Check sheet for the modelled part. Datum: model origin and axes. Units: mm. Face numbers are marked on the shaded views. A direction names the side the tool comes from. Give positions to 0.01 mm unless a question says otherwise; leave off trailing zeros. Write each loop counter-clockwise with the first axis right and the second up, starting at its lowest first coordinate (ties: lowest second). Pieces come first, ordered by that corner, then holes. Notation, with made-up numbers: (35.25, 1.25) -> (45.25, 1.25) arc R28 ccw to (45.25, 37.25) -> close; hole circle Ø5 at (74.25, -10). An arc over 180 degrees is marked (long way). Return JSON: item names as keys, results as strings.
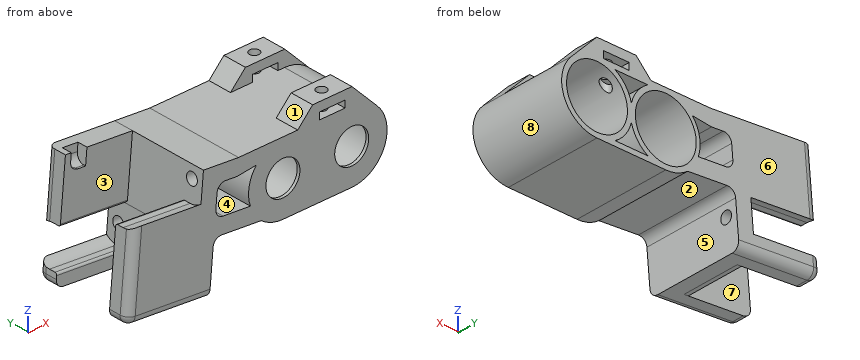
from build123d import *

# Parameters (mm, degrees)
SKETCH1_R               = 7.75
BOSS_EXTRUDE1_DEPTH     = 24
BOSS_EXTRUDE2_START     = 0.75
SKETCH2_R               = 4.33
BOSS_EXTRUDE2_DEPTH     = 0.75
SKETCH4_W               = 10
SKETCH4_H               = 6
BOSS_EXTRUDE4_DEPTH     = 4
CUT_EXTRUDE1_DEPTH      = 35.968736037
CUT_EXTRUDE1_DEPTH_BACK = 35.968736037
SKETCH5_W               = 6.5
SKETCH5_H               = 1.75
SKETCH6_R               = 1.25
CUT_EXTRUDE2_DEPTH      = 16
BOSS_EXTRUDE5_START     = -24.75
BOSS_EXTRUDE5_DEPTH     = 24.75
CUT_EXTRUDE3_DEPTH      = 39.520286863
SKETCH9_W               = 12.886425037
SKETCH9_H               = 24.75
BOSS_EXTRUDE6_DEPTH     = 4
FILLET1_R               = 2
FILLET2_R               = 2
BOSS_EXTRUDE9_DEPTH     = 17.13
SKETCH14_R              = 1.5
CUT_EXTRUDE5_DEPTH      = 6
BOSS_EXTRUDE10_DEPTH    = 14.84
FILLET4_R               = 2
SKETCH16_W              = 4
SKETCH16_H              = 2.5
CUT_EXTRUDE6_DEPTH      = 4
FILLET5_R               = 2
BOSS_EXTRUDE11_DEPTH    = 6
BOSS_EXTRUDE12_START    = -6
BOSS_EXTRUDE12_DEPTH    = 6


with BuildPart() as part:
    # Sketch1 → Boss-Extrude1 (new body)
    with BuildSketch(Plane(origin=(0, 0, 0), x_dir=(1, 0, 0), z_dir=(0, 1, 0))):
        with BuildLine():
            Line((0, -9), (17.5, -9))
            ThreePointArc((17.5, -9), (26.5, 0), (17.5, 9))
            Line((17.5, 9), (0, 9))
            ThreePointArc((0, 9), (-9, 0), (0, -9))
        make_face()
        with Locations(Location((17.5, 0, 0), (0, 0, 270))):
            Circle(SKETCH1_R, mode=Mode.SUBTRACT)
        with BuildLine():
            ThreePointArc((8.75, -2.106537443), (10.26424991, -5.352001554), (12.924248696, -7.75))
            Line((12.924248696, -7.75), (4.575751304, -7.75))
            ThreePointArc((4.575751304, -7.75), (7.23575009, -5.352001554), (8.75, -2.106537443))
        make_face(mode=Mode.SUBTRACT)
        with Locations(Location((0, 0, 0), (0, 0, 270))):
            Circle(SKETCH1_R, mode=Mode.SUBTRACT)
        with BuildLine():
            Line((4.575751304, 7.75), (12.924248696, 7.75))
            ThreePointArc((12.924248696, 7.75), (10.26424991, 5.352001554), (8.75, 2.106537443))
            ThreePointArc((8.75, 2.106537443), (7.23575009, 5.352001554), (4.575751304, 7.75))
        make_face(mode=Mode.SUBTRACT)
    extrude(amount=BOSS_EXTRUDE1_DEPTH)

    # Sketch2 → Boss-Extrude2 (add)
    with BuildSketch(Plane.XZ.offset(BOSS_EXTRUDE2_START)):
        with BuildLine():
            Line((17.5, 9), (0, 9))
            ThreePointArc((0, 9), (-9, 0), (0, -9))
            Line((0, -9), (17.5, -9))
            ThreePointArc((17.5, -9), (26.5, 0), (17.5, 9))
        make_face()
        with Locations(Location((17.5, 0, 0), (0, 0, 270))):
            Circle(SKETCH2_R, mode=Mode.SUBTRACT)
        with Locations(Location((0, 0, 0), (0, 0, 270))):
            Circle(SKETCH2_R, mode=Mode.SUBTRACT)
    extrude(amount=-BOSS_EXTRUDE2_DEPTH)

    # Sketch4 → Boss-Extrude4 (add)
    with BuildSketch(Plane.XY.offset(9)):
        with Locations((12.5625, 2.25)):
            Rectangle(SKETCH4_W, SKETCH4_H)
        with Locations((12.5625, 21)):
            Rectangle(SKETCH4_W, SKETCH4_H)
    extrude(amount=BOSS_EXTRUDE4_DEPTH)

    # Sketch5 → Cut-Extrude1 (cut, two sides: drawn at the far end of the back side and taken through both)
    with BuildSketch(Plane.XZ.offset(-18).offset(-CUT_EXTRUDE1_DEPTH_BACK)):
        with Locations((12.5625, 9.875)):
            Rectangle(SKETCH5_W, SKETCH5_H)
    extrude(amount=CUT_EXTRUDE1_DEPTH + CUT_EXTRUDE1_DEPTH_BACK, mode=Mode.SUBTRACT)

    # Sketch6 → Cut-Extrude2 (cut)
    with BuildSketch(Plane.XY.offset(13)):
        with Locations((12.5625, 2.25)):
            Circle(SKETCH6_R)
        with Locations((12.5625, 21)):
            Circle(SKETCH6_R)
    extrude(amount=-CUT_EXTRUDE2_DEPTH, mode=Mode.SUBTRACT)

    # Sketch7 → Boss-Extrude5 (add)
    with BuildSketch(Plane(origin=(0, 24, 0), x_dir=(1, 0, 0), z_dir=(0, 1, 0)).offset(BOSS_EXTRUDE5_START)):
        with BuildLine():
            Line((-20.224515403, -9.780709308), (-11.300967177, -9))
            Line((-11.300967177, -9), (0, -9))
            ThreePointArc((0, -9), (-8.505937794, -2.940922006), (-5.558955476, 7.077995056))
            Line((-5.558955476, 7.077995056), (-21.576855644, 5.676610378))
            Line((-21.576855644, 5.676610378), (-20.224515403, -9.780709308))
        make_face()
    extrude(amount=BOSS_EXTRUDE5_DEPTH)

    # Sketch8 → Cut-Extrude3 (cut, through all)
    with BuildSketch(Plane(origin=(0, 24, 0), x_dir=(1, 0, 0), z_dir=(0, 1, 0))):
        with BuildLine():
            Line((-16.588359581, -5.447307545), (-11.649590148, -5.015221208))
            Line((-11.649590148, -5.015221208), (-6.776158873, -5.535898385))
            ThreePointArc((-6.776158873, -5.535898385), (-8.611505528, -1.550636174), (-8.281582293, 2.824516725))
            Line((-8.281582293, 2.824516725), (-17.24345388, 2.040454557))
            Line((-17.24345388, 2.040454557), (-16.588359581, -5.447307545))
        make_face()
    extrude(amount=-CUT_EXTRUDE3_DEPTH, mode=Mode.SUBTRACT)

    # Sketch9 → Boss-Extrude6 (add)
    with BuildSketch(Plane(origin=(-20.92008866, 0, 1.830270598), x_dir=(0.08715574274765853, 0, 0.9961946980917455), z_dir=(-0.9961946980917455, 0, 0.08715574274765853))):
        with Locations((-13.978768561, 11.625)):
            Rectangle(SKETCH9_W, SKETCH9_H)
    extrude(amount=-BOSS_EXTRUDE6_DEPTH)

    # Fillet1
    fillet1_edges = [part.edges().sort_by_distance(p)[0] for p in [
        (-16.588359581, 11.625, 5.447307545),
        (-17.24345388, 11.625, -2.040454557),
        (-17.592076851, 11.625, -6.025233349),
    ]]
    fillet(fillet1_edges, radius=FILLET1_R)

    # Fillet2
    fillet2_edges = [part.edges().sort_by_distance(p)[0] for p in [
        (-20.707592193, -0.75, -18.688310163),
        (-20.707592193, 24, -18.688310163),
    ]]
    fillet(fillet2_edges, radius=FILLET2_R)

    # Sketch13 → Boss-Extrude9 (add)
    with BuildSketch(Plane(origin=(-20.92008866, 0, 1.830270598), x_dir=(0.08715574274765853, 0, 0.9961946980917455), z_dir=(-0.9961946980917455, 0, 0.08715574274765853))):
        with BuildLine():
            Line((-7.231981079, 21.08), (-7.231981079, 19.545))
            ThreePointArc((-7.231981079, 19.545), (-7.085534469, 19.191446609), (-6.731981079, 19.045))
            Line((-6.731981079, 19.045), (7.980808095, 19.045))
            Line((7.980808095, 19.045), (7.980808095, 24))
            Line((7.980808095, 24), (-8.270307829, 24))
            ThreePointArc((-8.270307829, 24), (-7.499287378, 22.629558198), (-7.231981079, 21.08))
        make_face()
        with BuildLine():
            Line((-20.421981079, 19.045), (-17.581981079, 19.045))
            ThreePointArc((-17.581981079, 19.045), (-17.228427688, 19.191446609), (-17.081981079, 19.545))
            Line((-17.081981079, 19.545), (-17.081981079, 21.08))
            ThreePointArc((-17.081981079, 21.08), (-16.814674779, 22.629558198), (-16.043654328, 24))
            Line((-16.043654328, 24), (-18.421981079, 24))
            ThreePointArc((-18.421981079, 24), (-19.836194641, 23.414213562), (-20.421981079, 22))
            Line((-20.421981079, 22), (-20.421981079, 19.045))
        make_face()
        with BuildLine():
            ThreePointArc((-0.281981079, 3.705), (-0.428427688, 4.058553391), (-0.781981079, 4.205))
            Line((-0.781981079, 4.205), (-20.421981079, 4.205))
            Line((-20.421981079, 4.205), (-20.421981079, 1.25))
            ThreePointArc((-20.421981079, 1.25), (-19.836194641, -0.164213562), (-18.421981079, -0.75))
            Line((-18.421981079, -0.75), (0.756345672, -0.75))
            ThreePointArc((0.756345672, -0.75), (-0.014674779, 0.620441802), (-0.281981079, 2.17))
            Line((-0.281981079, 2.17), (-0.281981079, 3.705))
        make_face()
    extrude(amount=BOSS_EXTRUDE9_DEPTH)

    # Sketch14 → Cut-Extrude5 (cut)
    with BuildSketch(Plane(origin=(-20.92008866, 0, 1.830270598), x_dir=(0.08715574274765853, 0, 0.9961946980917455), z_dir=(-0.9961946980917455, 0, 0.08715574274765853))):
        with Locations((-12.456981079, 21.08)):
            Circle(SKETCH14_R)
        with Locations((4.943018921, 2.17)):
            Circle(SKETCH14_R)
    extrude(amount=-CUT_EXTRUDE5_DEPTH, mode=Mode.SUBTRACT)

    # Sketch15 → Boss-Extrude10 (add)
    with BuildSketch(Plane.XZ.offset(-19.045)):
        with BuildLine():
            ThreePointArc((-22.605549661, -17.434636803), (-23.103926759, -18.03259557), (-23.779343463, -18.419566749))
            Line((-23.779343463, -18.419566749), (-22.699981589, -18.513998677))
            Line((-22.699981589, -18.513998677), (-22.605549661, -17.434636803))
        make_face()
    extrude(amount=BOSS_EXTRUDE10_DEPTH)

    # Fillet4
    fillet4_edges = [part.edges().sort_by_distance(p)[0] for p in [
        (-37.99751962, 24, 3.179049421),
        (-38.754734626, -0.75, -5.475957694),
        (-39.713742115, -0.164213562, -16.437463461),
        (-39.764796768, 2.7275, -17.021020804),
        (-39.764796768, 20.5225, -17.021020804),
        (-39.713742115, 23.414213562, -16.437463461),
        (-39.486842865, 24, -13.843993158),
    ]]
    fillet(fillet4_edges, radius=FILLET4_R)

    # Sketch16 → Cut-Extrude6 (cut)
    with BuildSketch(Plane(origin=(0.695573257, 0, 7.95043871), x_dir=(0.9961946980917455, 0, -0.08715574274765835), z_dir=(0.08715574274765836, 0, 0.9961946980917457))):
        with Locations((-34.63, 20.295)):
            Rectangle(SKETCH16_W, SKETCH16_H)
    extrude(amount=-CUT_EXTRUDE6_DEPTH, mode=Mode.SUBTRACT)

    # Fillet5
    fillet5_edges = [part.edges().sort_by_distance(p)[0] for p in [
        (-36.143661505, 20.295, 7.158174775),
        (-34.151272109, 21.545, 6.983863289),
    ]]
    fillet(fillet5_edges, radius=FILLET5_R)

    # Sketch17 → Boss-Extrude11 (add)
    with BuildSketch(Plane.XZ.offset(0.75)):
        Polygon((7.5625, 9), (7.5625, 13), (3.76173375, 9), align=None)
        with BuildLine():
            Line((24.024370778, 6.199402064), (17.5625, 13))
            Line((17.5625, 13), (17.5625, 9))
            Line((17.5625, 9), (17.5, 9))
            ThreePointArc((17.5, 9), (21.050026861, 8.270266579), (24.024370778, 6.199402064))
        make_face()
    extrude(amount=-BOSS_EXTRUDE11_DEPTH)

    # Sketch18 → Boss-Extrude12 (add)
    with BuildSketch(Plane(origin=(0, 24, 0), x_dir=(1, 0, 0), z_dir=(0, 1, 0)).offset(BOSS_EXTRUDE12_START)):
        with BuildLine():
            ThreePointArc((24.024370778, -6.199402064), (21.050026861, -8.270266579), (17.5, -9))
            Line((17.5, -9), (17.5625, -9))
            Line((17.5625, -9), (17.5625, -13))
            Line((17.5625, -13), (24.024370778, -6.199402064))
        make_face()
        Polygon((7.5625, -13), (7.5625, -9), (3.76173375, -9), align=None)
    extrude(amount=BOSS_EXTRUDE12_DEPTH)


solid = part.part
(1) Cross-section at A-A on x = -2. Enter the section's corners in (y, z), then the cut area to 3 significant figures.
Reply:
{"outline": "(-0.75, -8.77) -> (24, -8.77) -> (24, -7.49) -> (0, -7.49) -> (0, -3.84) -> (-0.75, -3.84) -> close; (-0.75, 3.84) -> (0, 3.84) -> (0, 7.49) -> (24, 7.49) -> (24, 9) -> (-0.75, 9) -> close", "area": "74.8 mm^2"}
(2) Depth check by flat-ended pin: pin 1 Ø0.7 at (x, z) = (-33.5, 10) entering from -Y (3 decimals); pin 2 Ø1.5 at (y, z) = (20, 8.5) entering from -X; pin 3 Ø1.5 at (x, y) = (12.56, 21) entering from +Z. Enter the tip coordinate at first touch or a pass-through.
Reply:
{"pin 1": "y = 21.545", "pin 2": "x = -37.6", "pin 3": "z = -5.26"}
(3) Release check for a two-part mould opening along Y. For the marked faces 5, 6, 7 and 8 record: pulls with the +Y half, pulls with the -Y half, needs draft (parallel to the pull), parting line crosses it, or undercut.
Reply:
{"face 5": "needs draft", "face 6": "pulls with the +Y half", "face 7": "undercut", "face 8": "undercut"}
(4) Set-up check for the marked faces 1, 2, 3 and 4: record each of +Z, -Z, +X, -X, +Y, -Y from which the full face is reachable in a straight line by a thin tool's end or side.
Reply:
{"face 1": "+Z, +Y, -Y", "face 2": "-Z, +Y, -Y", "face 3": "+Z, -X", "face 4": "+Y, -Y"}
(5) Thickness scan on L1, parallel to X at y = 11, z = 0; L2, parallel to Y at x = -23, z = 0.5 (3 decimals); L3, parallel to X at y = 19.25, z = 0. Record the ranges inside material, lowest first.
Reply:
{"L1": "-21.08 to -17.06, -8.75 to -7.75, 7.75 to 9.75, 25.25 to 26.5", "L2": "-0.75 to 4.205, 19.045 to 24", "L3": "-38.28 to -17.06, -8.75 to -7.75, 7.75 to 9.75, 25.25 to 26.5"}
(6) Cross-section at B-B on y = 13. Enter the section's corners in (x, z), then the cut area to 3 significant figures.
Reply:
{"outline": "(-23.78, -18.42) -> (-18.72, -18.86) -> (-17.77, -8.02) arc R2 cw to (-15.6, -6.2) -> (-5.56, -7.08) arc R9 ccw to (0, -9) -> (17.5, -9) arc R9 ccw to (17.5, 9) -> (-11.3, 9) -> (-20.22, 9.78) -> (-22.61, -17.43) arc R2.2 cw to start; hole (-17.07, -0.05) arc R2 ccw to (-15.25, -2.21) -> (-8.28, -2.82) arc R8.75 cw to (-6.78, 5.54) -> (-11.65, 5.02) -> (-14.6, 5.27) arc R2 ccw to (-16.76, 3.45) -> close; hole circle Ø15.5 at (0, 0); hole (4.58, -7.75) -> (12.92, -7.75) arc R9 cw to (8.75, -2.11) arc R9 cw to start; hole (4.58, 7.75) arc R9 cw to (8.75, 2.11) arc R9 cw to (12.92, 7.75) -> close; hole circle Ø15.5 at (17.5, 0)", "area": "357 mm^2"}
